Here's how the part is built. I have some questions about the finished solid (model axes, mm). A direction names the side the tool comes from. Round coordinates to 2 decimals unless told otherwise and drop trailing zeros. Loops run counter-clockwise (first coordinate to the right, second up) from the corner with the lowest first, then second, coordinate; pieces in that order, holes last. Notation, with made-up numbers: M 84,69.25 L 98,69.25 A22 cw 98,75.25 Z; hole C -2.75,14 d6. An arc over 180 degrees is marked long. Use a Markdown table: item, result.
```python
from build123d import *

# Parameters (mm, degrees)
SKETCH1_R                                            = 1.75
BOSS_EXTRUDE1_DEPTH                                  = 4
CSK_FOR_M3_HEX_SOCKET_COUNTERSUNK_CAP_SC_D           = 3.4
CSK_FOR_M3_HEX_SOCKET_COUNTERSUNK_CAP_SC_CSINK_D     = 6.72
CSK_FOR_M3_HEX_SOCKET_COUNTERSUNK_CAP_SC_CSINK_ANGLE = 90


with BuildPart() as part:
    # Sketch1 → Boss-Extrude1 (new body)
    with BuildSketch(Plane.XY):
        with BuildLine():
            Line((43.35, -60.5), (-43.35, -60.5))
            ThreePointArc((-43.35, -60.5), (-51.587794001, -57.087794001), (-55, -48.85))
            Line((-55, -48.85), (-55, 48.85))
            ThreePointArc((-55, 48.85), (-51.587794001, 57.087794001), (-43.35, 60.5))
            Line((-43.35, 60.5), (43.35, 60.5))
            ThreePointArc((43.35, 60.5), (51.587794001, 57.087794001), (55, 48.85))
            Line((55, 48.85), (55, -48.85))
            ThreePointArc((55, -48.85), (51.587794001, -57.087794001), (43.35, -60.5))
        make_face()
        with Locations((-47.488440649, 52.988440649)):
            Circle(SKETCH1_R, mode=Mode.SUBTRACT)
        with Locations(Location((47.488440649, 52.988440649, 0), (0, 0, 180))):
            Circle(SKETCH1_R, mode=Mode.SUBTRACT)
        with Locations((47.488440649, -52.988440649)):
            Circle(SKETCH1_R, mode=Mode.SUBTRACT)
        with Locations(Location((-47.488440649, -52.988440649, 0), (0, 0, 180))):
            Circle(SKETCH1_R, mode=Mode.SUBTRACT)
        with BuildLine():
            Line((39.4, -48.925), (-39.4, -48.925))
            ThreePointArc((-39.4, -48.925), (-42.228427125, -47.753427125), (-43.4, -44.925))
            Line((-43.4, -44.925), (-43.4, 44.925))
            ThreePointArc((-43.4, 44.925), (-42.228427125, 47.753427125), (-39.4, 48.925))
            Line((-39.4, 48.925), (39.4, 48.925))
            ThreePointArc((39.4, 48.925), (42.228427125, 47.753427125), (43.4, 44.925))
            Line((43.4, 44.925), (43.4, -44.925))
            ThreePointArc((43.4, -44.925), (42.228427125, -47.753427125), (39.4, -48.925))
        make_face(mode=Mode.SUBTRACT)
    extrude(amount=BOSS_EXTRUDE1_DEPTH)

    # CSK for M3 Hex Socket Countersunk Cap Screw1 (through all)
    with Locations(Plane.XY.offset(4)):
        with Locations((-47.488440649, -52.988440649), (47.488440649, -52.988440649), (47.488440649, 52.988440649), (-47.488440649, 52.988440649)):
            CounterSinkHole(CSK_FOR_M3_HEX_SOCKET_COUNTERSUNK_CAP_SC_D / 2, CSK_FOR_M3_HEX_SOCKET_COUNTERSUNK_CAP_SC_CSINK_D / 2, counter_sink_angle=CSK_FOR_M3_HEX_SOCKET_COUNTERSUNK_CAP_SC_CSINK_ANGLE)


solid = part.part
```
Q1. Imagine slicing it at D-D, the plane x = 47.5. Give the number of separate pieces and of enclosed holes in the cut face, then the cut area to 3 significant figures.
Return value:
| item | result |
|---|---|
| separate pieces | 3 |
| enclosed holes | 0 |
| area | 445 mm^2 |
Q2. For faces 1 (the conical face through (47.9, -54.8, 2.5)), 2 (the cylindrical face through (42.26, -47.72, 1.97)), which set-ups out of +Z, -Z, +X, -X, +Y, -Y let a thin tool reach every point of the face, with its end or its side?
Return value:
| item | result |
|---|---|
| face 1 | +Z |
| face 2 | +Z, -Z |
Q3. Imagine slicing it at A-A, the plane y = -18.5. Please give me the cut outline in (x, z).
Return value:
| item | result |
|---|---|
| outline | M -55,0 L -43.4,0 L -43.4,4 L -55,4 Z; M 43.4,0 L 55,0 L 55,4 L 43.4,4 Z |
Q4. We'd pull the mould along Y, two halves only. Please class faces 3 (the cylindrical face through (42.2, 47.78, 1.97)), 4 (the cylindrical face through (-51.678, 56.997, 1.972)), 5 (the flat face through (45, -4, 4)): pulls with the +Y half, pulls with the -Y half, needs draft (parallel to the pull), parting line crosses it, or undercut.
Return value:
| item | result |
|---|---|
| face 3 | undercut |
| face 4 | pulls with the +Y half |
| face 5 | needs draft |
Q5. Imagine slicing it at C-C, the plane z = 1.65. Please give me the cut outline in (x, y) (3 decimals), then the cut area to 3 significant figures.
Return value:
| item | result |
|---|---|
| outline | M -55,-48.85 A11.65 ccw -43.35,-60.5 L 43.35,-60.5 A11.65 ccw 55,-48.85 L 55,48.85 A11.65 ccw 43.35,60.5 L -43.35,60.5 A11.65 ccw -55,48.85 Z; hole C -47.488,-52.988 d3.5; hole C -47.488,52.988 d3.5; hole M -43.4,-44.925 A4 ccw -39.4,-48.925 L 39.4,-48.925 A4 ccw 43.4,-44.925 L 43.4,44.925 A4 ccw 39.4,48.925 L -39.4,48.925 A4 ccw -43.4,44.925 Z; hole C 47.488,-52.988 d3.5; hole C 47.488,52.988 d3.5 |
| area | 4,680 mm^2 |
Q6. Will these pins go through, and if not, where does the flat tip stop? P1, Ø12, axis at x = -10.5, y = -39.5, coming from the -Z side; P2, Ø4.5, axis at x = -47.49, y = 52.99, coming from the -Z side; P3, Ø4, axis at x = 47.49, y = 52.99, coming from the +Z side.
Return value:
| item | result |
|---|---|
| P1 | passes through |
| P2 | stops at z = 0 |
| P3 | stops at z = 2.64 |
Q7. Imagine slicing it at B-B, the plane x = -38. Please give me the cut outline in (y, z) (3 decimals).
Return value:
| item | result |
|---|---|
| outline | M -60.5,0 L -48.925,0 L -48.925,4 L -60.5,4 Z; M 48.925,0 L 60.5,0 L 60.5,4 L 48.925,4 Z |
Q8. I need wall thicknesses on line 1 (Y direction, x = -17.5, z = 1.8) (3 decimals); line 2 (X direction, y = -41.5, z = 2.5); line 3 (Y direction, x = -43, z = 2.55). Which ranges of each line are inside material? Lowest first, please. Write a range as from..to.
Return value:
| item | result |
|---|---|
| line 1 | y = -60.5..-48.925, 48.925..60.5 |
| line 2 | x = -55..-43.4, 43.4..55 |
| line 3 | y = -60.5..-46.67, 46.67..60.5 |
